Read the model definition and answer for the solid it produces. Units are mm, in the model's axes. A direction names the side the tool comes from. Round coordinates to 2 decimals unless told otherwise and drop trailing zeros. Order: outer loops, then holes, each group sorted by start corner. A loop starts at its lowest first (then second) coordinate and runs counter-clockwise, first axis right, second up. Notation, with made-up numbers: (-5, 37.5) - (42, 37.5) arc R17 cw to (42, 63.5) - close; hole circle Ø8 at (37.25, 30). An arc over 180 degrees is marked (long way). Answer as a JSON object with one key per item and string values. Group by question number.
Q1. The mould has two halves that part along Y. Classify faces 3 (the cylindrical face through (11.9, 16.5, 15.1)), 4 (the flat face through (21, 3.8, 30)), 5 (the flat face through (33.24, 6.887, 14.79)), 6 (the flat face through (8.5, 0.5, 14.8)): pulls with the +Y half, pulls with the -Y half, needs draft (parallel to the pull), parting line crosses it, or undercut.
Q2. A cutting plane is placed at C-C on z = 19.25. Determine the outline of the cut face in (x, y).
Q3. Given pin 1 Ø13 at (x, z) = (13.5, 12) entering from -Y; pin 2 Ø3.5 at (x, z) = (29.5, 24.5) entering from -Y; pin 3 Ø5 at (y, z) = (14.5, 17.5) entering from -X; pin 4 Ø3.5 at (x, z) = (4.5, 5.5) entering from +Y, each flat-ended and moving along its own axis, determine where each tip first touches the part or whether it passes through.
Q4. A tool of negligible diameter and unlimited length cuts with its end or side. For faces 1 (the flat face through (21, 4, 0)), 2 (the flat face through (17, 1, 15)), from which of +Z, -Z, +X, -X, +Y, -Y can it reach the whole face along a straight path? Write none if from no direction.
Q5. A cutting plane is placed at B-B on x = 29.5. Determine the outline of the cut face in (y, z), and give its area (3 significant figures).
Q6. Consider line 1 (Z direction, x = 29.5, y = 10.5); line 2 (Z direction, x = 5.5, y = 5); line 3 (X direction, y = 9, z = 5.5). Determine where each line is inside the solid, lowest interval first.
Q7. A cutting plane is placed at A-A on z = 24.5. Count the separate pieces of the cut face and the enclosed holes in it, and give its area (3 significant figures).
```python
from build123d import *

# Parameters (mm, degrees)
BOSS_EXTRUDE1_DEPTH        = 30
M5_TAPPED_HOLE5_AT_2_COUNT = 2
M5_TAPPED_HOLE5_AT_2_PITCH = 19
M5_TAPPED_HOLE6_AT_2_COUNT = 2
M5_TAPPED_HOLE6_AT_2_PITCH = 19


with BuildPart() as part:
    # Sketch1 → Boss-Extrude1 (new body)
    with BuildSketch(Plane.XY):
        Polygon((0, 0), (0, 6), (1.5, 7.75), (1.5, 17.75), (9.5, 17.75), (13.5, 21.75), (20.5, 21.75), (24.5, 17.75), (32.5, 17.75), (32.5, 7.75), (34, 6), (34, 0), (26, 0), (25, 1), (9, 1), (8, 0), align=None)
    extrude(amount=BOSS_EXTRUDE1_DEPTH)

    # Sketch4 → CSK for M5 Countersunk Flat Head Screw1 (revolve, cut)
    with BuildSketch(Plane(origin=(17, 11, 30), x_dir=(0, -1, 0), z_dir=(1, 0, 0))):
        Polygon((0, 0), (0, 30), (7.75, 30), (7.5, 29.75), (7.5, 0.5), (8, 0), align=None)
    revolve(axis=Axis((17, 11, 36.35), (0, 0, -1)), mode=Mode.SUBTRACT)

    # Sketch19 → M5 Tapped Hole5 (revolve, cut)
    with BuildSketch(Plane(origin=(29.5, 0, 5.5), x_dir=(0, 0, -1), z_dir=(1, 0, 0))):
        Polygon((0, 0), (0, 17.75), (2.5, 17.75), (1.5, 16.75), (1.5, 1), (2.5, 0), align=None)
    m5_tapped_hole5 = revolve(axis=Axis((29.5, -6.35, 5.5), (0, 1, 0)), mode=Mode.SUBTRACT)

    # M5 Tapped Hole5 at 2: M5 Tapped Hole5 ×2
    with Locations(*[(0, 0, i * M5_TAPPED_HOLE5_AT_2_PITCH) for i in range(1, M5_TAPPED_HOLE5_AT_2_COUNT)]):
        add(m5_tapped_hole5, mode=Mode.SUBTRACT)

    # Sketch21 → M5 Tapped Hole6 (revolve, cut)
    with BuildSketch(Plane(origin=(4.5, 0, 5.5), x_dir=(0, 0, -1), z_dir=(1, 0, 0))):
        Polygon((0, 0), (0, 17.75), (2.5, 17.75), (1.5, 16.75), (1.5, 1), (2.5, 0), align=None)
    m5_tapped_hole6 = revolve(axis=Axis((4.5, -6.35, 5.5), (0, 1, 0)), mode=Mode.SUBTRACT)

    # M5 Tapped Hole6 at 2: M5 Tapped Hole6 ×2
    with Locations(*[(0, 0, i * M5_TAPPED_HOLE6_AT_2_PITCH) for i in range(1, M5_TAPPED_HOLE6_AT_2_COUNT)]):
        add(m5_tapped_hole6, mode=Mode.SUBTRACT)


solid = part.part
```
Result set:
{
 "1": {"face 3": "undercut", "face 4": "needs draft", "face 5": "pulls with the +Y half", "face 6": "pulls with the -Y half"},
 "2": {"outline": "(0, 0) - (8, 0) - (9, 1) - (25, 1) - (26, 0) - (34, 0) - (34, 6) - (32.5, 7.75) - (32.5, 17.75) - (24.5, 17.75) - (20.5, 21.75) - (13.5, 21.75) - (9.5, 17.75) - (1.5, 17.75) - (1.5, 7.75) - (0, 6) - close; hole circle Ø15 at (17, 11)"},
 "3": {"pin 1": "stops at y = 0", "pin 2": "stops at y = 0.75", "pin 3": "stops at x = 1.5", "pin 4": "stops at y = 17"},
 "4": {"face 1": "-Z, +X, -X, +Y, -Y", "face 2": "+Z, -Z, -Y"},
 "5": {"outline": "(0, 0) - (17.75, 0) - (17.75, 3) - (16.75, 4) - (1, 4) - (0, 3) - close; (0, 8) - (1, 7) - (16.75, 7) - (17.75, 8) - (17.75, 22) - (16.75, 23) - (1, 23) - (0, 22) - close; (0, 27) - (1, 26) - (16.75, 26) - (17.75, 27) - (17.75, 30) - (0, 30) - close", "area": "422 mm²"},
 "6": {"line 1": "z = 0 to 4, 7 to 23, 26 to 30", "line 2": "z = 0 to 4.38, 6.62 to 23.38, 25.62 to 30", "line 3": "x = 1.5 to 3, 6 to 9.77, 24.23 to 28, 31 to 32.5"},
 "7": {"separate pieces": "3", "enclosed holes": "1", "area": "311 mm²"}
}
